The listing builds one solid part. Answer for the finished solid, in the listing's coordinates (mm). Face numbers are marked on the shaded views. Coordinates: 2 decimals unless noted, no trailing zeros. Loops run counter-clockwise (first coordinate to the right, second up) from the corner with the lowest first, then second, coordinate; pieces in that order, holes last. Notation, with made-up numbers: (-30.75, -35.75) - (-1.75, -35.75) arc R20 ccw to (-1.75, -17.75) - close; hole circle Ø8 at (40.5, -28.75). An arc over 180 degrees is marked (long way). Put each result on its own line as item: value.
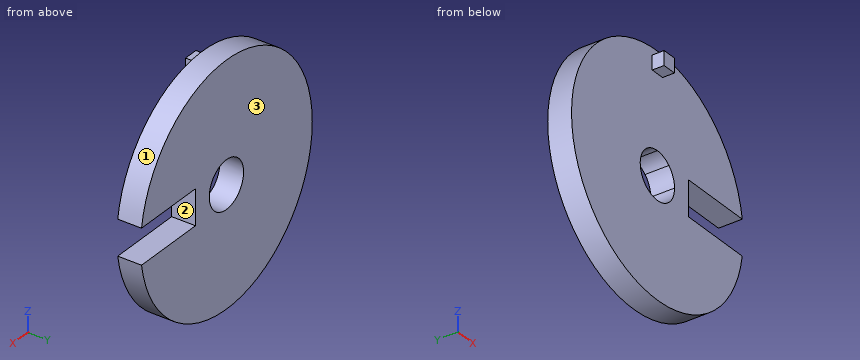
```python
from build123d import *

# Parameters (mm, degrees)
F0_W     = 30
F0_H     = 60
F1_DEPTH = 100
F2_DEPTH = 102
F4_DEPTH = 100
F5_DEPTH = 150


# Not quite as in the source:
# - a feature of the source that left no trace in its solid (it failed there, or was rolled back) is left out
# - a feature names something its author has since deleted; it is built from what else it names


with BuildPart() as f1:
    # F0 (on Front) → F1 (new body)
    with BuildSketch(Plane.XZ):
        with BuildLine():
            Line((180.2002936602, 74.2409452796), (494.457563441, 74.2409452796))
            ThreePointArc((494.457563441, 74.2409452796), (326.2510746037, 378.8934366282), (0, 500))
            Line((0, 500), (0, 468.3614957333))
            Line((0, 468.3614957333), (30, 468.3614957333))
            Line((30, 468.3614957333), (30, 408.3614957333))
            Line((30, 408.3614957333), (0, 408.3614957333))
            Line((0, 408.3614957333), (0, 100))
            ThreePointArc((0, 100), (35.8880584042, 93.3383483033), (66.9946419051, 74.2409452796))
            Line((66.9946419051, 74.2409452796), (180.2002936602, 74.2409452796))
        make_face()
        with BuildLine():
            ThreePointArc((0, 500), (-378.8934366282, -326.2510746037), (494.457563441, -74.2409452796))
            Line((494.457563441, -74.2409452796), (180.2002936602, -74.2409452796))
            Line((180.2002936602, -74.2409452796), (66.9946419051, -74.2409452796))
            ThreePointArc((66.9946419051, -74.2409452796), (-93.3383483033, -35.8880584042), (0, 100))
            Line((0, 100), (0, 408.3614957333))
            Line((0, 408.3614957333), (-30, 408.3614957333))
            Line((-30, 408.3614957333), (-30, 468.3614957333))
            Line((-30, 468.3614957333), (0, 468.3614957333))
            Line((0, 468.3614957333), (0, 500))
        make_face()
        with BuildLine():
            Line((180.2002936602, -74.2409452796), (180.2002936602, 74.2409452796))
            Line((180.2002936602, 74.2409452796), (66.9946419051, 74.2409452796))
            ThreePointArc((66.9946419051, 74.2409452796), (91.3768684912, 40.6234895688), (100, 0))
            ThreePointArc((100, 0), (91.3768684912, -40.6234895688), (66.9946419051, -74.2409452796))
            Line((66.9946419051, -74.2409452796), (180.2002936602, -74.2409452796))
        make_face()
        with Locations((-15, 438.3614957333)):
            Rectangle(F0_W, F0_H)
    extrude(amount=F1_DEPTH)

    # F0 (on Front) → F2 (join)
    with BuildSketch(Plane.XZ):
        with Locations((15, 438.3614957333)):
            Rectangle(F0_W, F0_H)
    extrude(amount=F2_DEPTH)

    # F0 (on Front) → F4 (join)
    with BuildSketch(Plane.XZ):
        with BuildLine():
            Line((180.2002936602, 74.2409452796), (494.457563441, 74.2409452796))
            ThreePointArc((494.457563441, 74.2409452796), (326.2510746037, 378.8934366282), (0, 500))
            Line((0, 500), (0, 468.3614957333))
            Line((0, 468.3614957333), (30, 468.3614957333))
            Line((30, 468.3614957333), (30, 408.3614957333))
            Line((30, 408.3614957333), (0, 408.3614957333))
            Line((0, 408.3614957333), (0, 100))
            ThreePointArc((0, 100), (35.8880584042, 93.3383483033), (66.9946419051, 74.2409452796))
            Line((66.9946419051, 74.2409452796), (180.2002936602, 74.2409452796))
        make_face()
    extrude(amount=F4_DEPTH)

    # F0 (on Front) → F5 (join)
    with BuildSketch(Plane.XZ):
        with Locations((-15, 438.3614957333)):
            Rectangle(F0_W, F0_H)
        with Locations((15, 438.3614957333)):
            Rectangle(F0_W, F0_H)
    extrude(amount=F5_DEPTH)


solid = f1.part
```
1) The part is cut by section A-A (y = -48). Give the vertices of the cut face in (x, z), and give its area (3 significant figures).
Found:
outline: (180.2, -74.24) - (180.2, 74.24) - (494.46, 74.24) arc R500 ccw (long way) to (494.46, -74.24) - close; hole circle Ø200 at (0, 0)
area: 707,000 mm^2
2) Each of these flat-tipped pins is pushed along its axis until it touches: pin 1 (1.5 mm diameter, centred on y = -23, z = -170.5, fed in from +X); pin 2 (8 mm diameter, centred on y = -97.5, z = 58.5, fed in from -X); pin 3 (8 mm diameter, centred on x = -143, z = -155, fed in from -Y). Where does it stop, or does it pass through?
Found:
pin 1: stops at x = 470.3
pin 2: stops at x = -497.02
pin 3: stops at y = -100
3) The part is cut by section B-B (x = -62). Give the vertices of the cut face in (y, z), and give its area (3 significant figures).
Found:
outline: (-100, -496.14) - (0, -496.14) - (0, -78.46) - (-100, -78.46) - close; (-100, 78.46) - (0, 78.46) - (0, 496.14) - (-100, 496.14) - close
area: 83,500 mm^2
4) For a pull along Z with two mould halves and no side action, classify the marked faces 1, 2 and 3 as pulls with the +Z half, pulls with the -Z half, needs draft (parallel to the pull), parting line crosses it, or undercut.
Found:
face 1: parting line crosses it
face 2: undercut
face 3: needs draft
5) The part is cut by section C-C (z = 436.5). Give the vertices of the cut face in (x, y), and give its area (3 significant figures).
Found:
outline: (-243.86, -100) - (-30, -100) - (-30, -150) - (30, -150) - (30, -100) - (243.86, -100) - (243.86, 0) - (-243.86, 0) - close
area: 51,800 mm^2
6) Straight lines are drawn through the part: L1, parallel to Z at x = 0, y = -36.5; L2, parallel to Y at x = -160, z = -283; L3, parallel to Z at x = 238.5, y = -44.5. For each, find the intervals that lie inside material, in ascending order. Write a range as [from, to].
Found:
L1: z = [-500, -100], [100, 500]
L2: y = [-100, 0]
L3: z = [-439.45, -74.24], [74.24, 439.45]
7) The part is cut by section D-D (x = 391). Give the vertices of the cut face in (y, z).
Found:
outline: (-100, -311.64) - (0, -311.64) - (0, -74.24) - (-100, -74.24) - close; (-100, 74.24) - (0, 74.24) - (0, 311.64) - (-100, 311.64) - close
